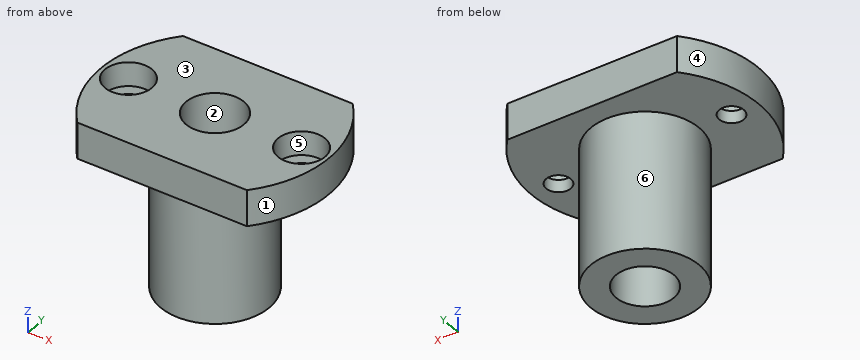
from build123d import *

# Parameters (mm, degrees)
SKETCH1_R           = 7.5
SKETCH1_R_2         = 1.7
SKETCH1_R_3         = 4
BOSS_EXTRUDE1_DEPTH = 5
BOSS_EXTRUDE2_START = -19
SKETCH1_3_R         = 7.5
SKETCH1_3_R_2       = 4
BOSS_EXTRUDE2_DEPTH = 19
SKETCH2_R           = 3.25
CUT_EXTRUDE1_DEPTH  = 3.3


with BuildPart() as part:
    # Sketch1 → Boss-Extrude1 (new body)
    # profile 1 of 2: a face of its own
    with BuildSketch(Plane.XY):
        with BuildLine():
            Line((-11.760078621, -10.5), (11.760078621, -10.5))
            ThreePointArc((11.760078621, -10.5), (15.765451125, 0), (11.760078621, 10.5))
            Line((11.760078621, 10.5), (-11.760078621, 10.5))
            ThreePointArc((-11.760078621, 10.5), (-15.765451125, 0), (-11.760078621, -10.5))
        make_face()
        Circle(SKETCH1_R, mode=Mode.SUBTRACT)
        with Locations((-12, 0)):
            Circle(SKETCH1_R_2, mode=Mode.SUBTRACT)
        with Locations((12, 0)):
            Circle(SKETCH1_R_2, mode=Mode.SUBTRACT)
    # profile 2 of 2: a face of its own
    with BuildSketch(Plane.XY):
        Circle(SKETCH1_R)
        Circle(SKETCH1_R_3, mode=Mode.SUBTRACT)
    extrude(amount=BOSS_EXTRUDE1_DEPTH)

    # Sketch1_3 → Boss-Extrude2 (add)
    with BuildSketch(Plane.XY.offset(BOSS_EXTRUDE2_START)):
        Circle(SKETCH1_3_R)
        Circle(SKETCH1_3_R_2, mode=Mode.SUBTRACT)
    extrude(amount=BOSS_EXTRUDE2_DEPTH)

    # Sketch2 → Cut-Extrude1 (cut)
    with BuildSketch(Plane.XY.offset(5)):
        with Locations((-12, 0)):
            Circle(SKETCH2_R)
        with Locations(Location((12, 0, 0), (0, 0, 180))):
            Circle(SKETCH2_R)
    extrude(amount=-CUT_EXTRUDE1_DEPTH, mode=Mode.SUBTRACT)


solid = part.part
Source: CAD feature listing. Evaluate the final solid. Frame: model axes, mm. Face numbers are marked on the shaded views. A direction names the side the tool comes from. Round coordinates to 2 decimals unless told otherwise and drop trailing zeros. Loops run counter-clockwise (first coordinate to the right, second up) from the corner with the lowest first, then second, coordinate; pieces in that order, holes last.
Q1. Mould query, pull axis X, two halves, no side actions, for the marked faces 1, 2 and 3. Classes: pulls with the +X half, pulls with the -X half, needs draft (parallel to the pull), parting line crosses it, or undercut.
Q2. Access query for the marked faces 4, 5 and 6. Directions: +Z, -Z, +X, -X, +Y, -Y. A direction counts if a zero-diameter tool reaches every point of the face in a straight line with its end or side. Return the directions, or none.
Q3. Ray query, line 1 (X direction, y = 1, z = 2.5); line 2 (Z direction, x = 3, y = -7.5); line 3 (Z direction, x = -10, y = 1.25). Return the intervals inside material, ascending.
Q4. Section B-B, the plane z = 3. Return loops of the section in (x, y), plus the area to 3 significant figures.
Q5. Section A-A, the plane y = 0. Return loops of the section in (x, z), plus the area to 3 significant figures.
Q6. Section D-D, the plane y = 2.75. Return loops of the section in (x, z).
Q7. Section C-C, the plane x = 0. Return loops of the section in (y, z), plus the area to 3 significant figures.
Q8. First-contact query: P1, Ø1, axis at y = 7, z = -11, coming from the -X side; P2, Ø5.5, axis at x = -12, y = 0, coming from the -Z side; P3, Ø1.5, axis at y = 3, z = -6, coming from the -X side. Flat tips, straight axial feed; report the tip coordinate or a pass-through.
Solutions:
1. face 1: pulls with the +X half
1. face 2: undercut
1. face 3: needs draft
2. face 4: +Z, -Z, -X
2. face 5: +Z
2. face 6: -Z
3. line 1: x = -15.73 to -15.09, -8.91 to -3.87, 3.87 to 8.91, 15.09 to 15.73
3. line 2: z = 0 to 5
3. line 3: z = 0 to 1.7
4. outline: (-11.76, -10.5) - (11.76, -10.5) arc R15.77 ccw to (11.76, 10.5) - (-11.76, 10.5) arc R15.77 ccw to start; hole circle Ø6.5 at (-12, 0); hole circle Ø8 at (0, 0); hole circle Ø6.5 at (12, 0)
4. area: 493 mm2
5. outline: (-15.77, 0) - (-13.7, 0) - (-13.7, 1.7) - (-15.25, 1.7) - (-15.25, 5) - (-15.77, 5) - close; (-10.3, 0) - (-7.5, 0) - (-7.5, -19) - (-4, -19) - (-4, 5) - (-8.75, 5) - (-8.75, 1.7) - (-10.3, 1.7) - close; (4, -19) - (7.5, -19) - (7.5, 0) - (10.3, 0) - (10.3, 1.7) - (8.75, 1.7) - (8.75, 5) - (4, 5) - close; (13.7, 0) - (15.77, 0) - (15.77, 5) - (15.25, 5) - (15.25, 1.7) - (13.7, 1.7) - close
5. area: 196 mm2
6. outline: (-15.52, 0) - (-6.98, 0) - (-6.98, -19) - (-2.9, -19) - (-2.9, 5) - (-10.27, 5) - (-10.27, 1.7) - (-13.73, 1.7) - (-13.73, 5) - (-15.52, 5) - close; (2.9, -19) - (6.98, -19) - (6.98, 0) - (15.52, 0) - (15.52, 5) - (13.73, 5) - (13.73, 1.7) - (10.27, 1.7) - (10.27, 5) - (2.9, 5) - close
7. outline: (-10.5, 0) - (-7.5, 0) - (-7.5, -19) - (-4, -19) - (-4, 5) - (-10.5, 5) - close; (4, -19) - (7.5, -19) - (7.5, 0) - (10.5, 0) - (10.5, 5) - (4, 5) - close
7. area: 198 mm2
8. P1: stops at x = -3.74
8. P2: stops at z = 0
8. P3: stops at x = -7.15
